Source: CAD feature listing. Evaluate the final solid. Frame: model axes, mm. A direction names the side the tool comes from. Give positions to 0.01 mm unless a question says otherwise; leave off trailing zeros. Loops run counter-clockwise (first coordinate to the right, second up) from the corner with the lowest first, then second, coordinate; pieces in that order, holes last. Notation, with made-up numbers: M 22.25,85.5 L 49.25,85.5 A9 cw 49.25,93.5 Z; hole C 24.25,47.25 d7. An arc over 180 degrees is marked long. Write item = value, one per line.
from build123d import *

# Parameters (mm, degrees)
F0_R     = 25.7
F0_R_2   = 25
F0_R_3   = 4.05
F1_DEPTH = 9.16
F3_W     = 136.57
F3_H     = 51.4
F4_DEPTH = 9.16
F2_R     = 25
F2_R_2   = 4.05
F5_DEPTH = 9
F6_DEPTH = 25
F7_W     = 25.7
F7_H     = 74.087158006
F7_H_2   = 74.0871579793
F8_DEPTH = 25
F9_DEPTH = 1


with BuildPart() as f1:
    # F0 (on Top) → F1 (new body)
    with BuildSketch(Plane.XY):
        Circle(F0_R)
        Circle(F0_R_2, mode=Mode.SUBTRACT)
        Circle(F0_R_2)
        with Locations((13.04, 10.1912168066)):
            Circle(F0_R_3, mode=Mode.SUBTRACT)
    extrude(amount=F1_DEPTH)



with BuildPart() as f1b:
    # F0 (on Top) → F1, piece 2 (new body)
    with BuildSketch(Plane.XY):
        with Locations((136.57, 0)):
            Circle(F0_R)
        with Locations((136.57, 0)):
            Circle(F0_R_2, mode=Mode.SUBTRACT)
        with Locations((136.57, 0)):
            Circle(F0_R_2)
        with Locations((123.53, 10.1912168066)):
            Circle(F0_R_3, mode=Mode.SUBTRACT)
    extrude(amount=F1_DEPTH)


with BuildPart() as f1_1:
    add(f1.part)

    add(f1b.part)  # F4 merges F1b
    # F3 (on Top) → F4 (join)
    with BuildSketch(Plane.XY):
        with Locations((68.285, 0)):
            Rectangle(F3_W, F3_H)
    extrude(amount=F4_DEPTH)

    # F2 (on Top) → F5 (cut)
    with BuildSketch(Plane.XY):
        Circle(F2_R)
        with Locations((13.04, 10.1912168066)):
            Circle(F2_R_2, mode=Mode.SUBTRACT)
        with Locations((136.57, 0)):
            Circle(F2_R)
        with Locations((123.53, 10.1912168066)):
            Circle(F2_R_2, mode=Mode.SUBTRACT)
    extrude(amount=F5_DEPTH, mode=Mode.SUBTRACT)

    # F6 (cut): faces of the model
    f6_faces = [f1_1.faces().sort_by_distance(p)[0] for p in [
        (123.53, 10.1912168066, 0),
        (13.04, 10.1912168066, 0),
    ]]
    extrude(f6_faces, amount=-F6_DEPTH, mode=Mode.SUBTRACT)

    # F7 (on Top) → F8 (cut)
    with BuildSketch(Plane.XY):
        with Locations((-12.85, -2.68e-08)):
            Rectangle(F7_W, F7_H)
        with Locations((149.42, 1.34e-08)):
            Rectangle(F7_W, F7_H_2)
    extrude(amount=F8_DEPTH, mode=Mode.SUBTRACT)

    # F9 (add): a face of the model
    f9_faces = [f1_1.faces().sort_by_distance(p)[0] for p in [
        (68.285, -0.1518521362, 9.16),
    ]]
    extrude(f9_faces, amount=F9_DEPTH)


solid = f1_1.part
1. First-contact query: pin 1 Ø10.5 at (x, y) = (123.53, 10.19) entering from -Z; pin 2 Ø2 at (y, z) = (-17.5, 2) entering from +X; pin 3 Ø2 at (y, z) = (-8, 3) entering from -X. Flat tips, straight axial feed; report the tip coordinate or a pass-through.
Derived:
pin_1 = 9
pin_2 = 119.75
pin_3 = 23.32
2. Material intervals for probe 1 along X at (y, z) = (10.5, 9.75); probe 2 along Y at (x, z) = (13.04, 9.8); probe 3 along Y at (x, z) = (16.5, 3), sorted ascending. Write a range as from..to.
Derived:
probe_1 = 0..9, 17.08..119.49, 127.57..136.57
probe_2 = -25.7..6.14, 14.24..25.7
probe_3 = -25.7..-18.78, 18.78..25.7
3. Reachability of faces 1 (the flat face through (10, 0, 9)), 2 (the flat face through (136.57, 0, 10)), 3 (the cylindrical face through (111.576, 0.55, 4.437)) from +Z, -Z, +X, -X, +Y, -Y: full face, straight path, thin tool, end or side. Return the list, or none.
Derived:
face_1 = -Z, -X
face_2 = +Z, -Z, +X, +Y, -Y
face_3 = -Z, +X
4. Cut plane B-B, the plane y = 11.5. Return the cut outline in (x, z).
Derived:
outline = M 0,9 L 9.21,9 L 9.21,10.16 L 0,10.16 Z; M 16.87,9 L 22.2,9 L 22.2,0 L 114.37,0 L 114.37,9 L 119.7,9 L 119.7,10.16 L 16.87,10.16 Z; M 127.36,9 L 136.57,9 L 136.57,10.16 L 127.36,10.16 Z
5. Cut plane D-D, the plane y = 0. Return the cut outline in (x, z), then the cut area to 3 significant figures.
Derived:
outline = M 0,9 L 25,9 L 25,0 L 111.57,0 L 111.57,9 L 136.57,9 L 136.57,10.16 L 0,10.16 Z
area = 938 mm²
6. Cut plane C-C, the plane x = 13.04. Return the cut outline in (y, z).
Derived:
outline = M -25.7,0 L -21.33,0 L -21.33,9 L 6.14,9 L 6.14,10.16 L -25.7,10.16 Z; M 14.24,9 L 21.33,9 L 21.33,0 L 25.7,0 L 25.7,10.16 L 14.24,10.16 Z
7. Pull-direction query (Y, two-part tool) for faces 4 (the flat face through (67, 0, 0)), 5 (the cylindrical face through (24.994, -0.55, 4.437)), 6 (the flat face through (67, 25.7, 5)), 7 (the cylindrical face through (12.16, 6.24, 9.57)); classes: +Y half, -Y half, draft (parallel to the pull), parting line (faces both ways), or undercut.
Derived:
face_4 = draft
face_5 = undercut
face_6 = +Y half
face_7 = undercut
8. Cut plane A-A, the plane z = 1.25. Return the cut outline in (x, y).
Derived:
outline = M 0,-25.7 L 136.57,-25.7 L 136.57,-25 A25 cw 136.57,25 L 136.57,25.7 L 0,25.7 L 0,25 A25 cw 0,-25 Z
